Study the drawing (mm; zero at the part's minimum x, y, z) and answer. A direction names the side the tool comes from. Give positions to 0.01 mm unless a question says otherwise; leave off trailing zeros. Order: outer loops, then holes, each group sorted by start corner. A loop starts at its lowest first (then second) coordinate and runs counter-clockwise, first axis right, second up. Notation, with made-up numbers: (41, -37) - (83, -37) arc R10 cw to (83, -25) - close; hole circle Ø8 at (34, 83.5). An arc over 180 degrees is marked (long way). Use CSV: the item, a comma, the result in double quotes.
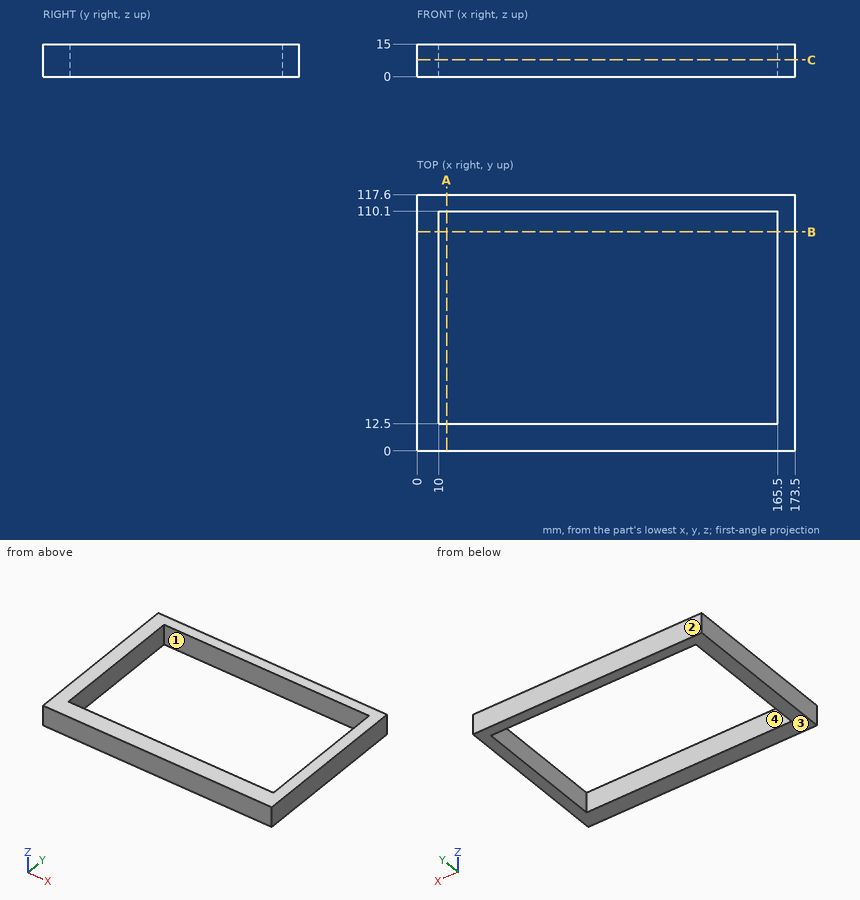
Item 1: Which of the six approach directions +Z, -Z, +X, -X, +Y, -Y give full straight-line access (tool end or side, diameter ignored) to the marked faces 3 and 4?
Taken from the geometry:
face 3,"-Z, +X, -X, +Y, -Y"
face 4,"+Z, -Z"
Item 2: The part is cut by section A-A (x = 13.5). Give the vertices of the cut face in (y, z).
Taken from the geometry:
outline,"(0, 0) - (12.5, 0) - (12.5, 15) - (0, 15) - close; (110.1, 0) - (117.6, 0) - (117.6, 15) - (110.1, 15) - close"
Item 3: The part is cut by section C-C (z = 7.75). Give the vertices of the cut face in (x, y), and give its area (3 significant figures).
Taken from the geometry:
outline,"(0, 0) - (173.5, 0) - (173.5, 117.6) - (0, 117.6) - close; hole (10, 12.5) - (165.5, 12.5) - (165.5, 110.1) - (10, 110.1) - close"
area,"5,230 mm^2"
Item 4: This flat-tipped pin is pushed along its axis until it touches: pin 1 (12 mm diameter, centred on x = 18, y = 89, fed in from +Z) (3 decimals). Where does it stop, or does it pass through?
Taken from the geometry:
pin 1,"through"
Item 5: Find the intervals of material crossed by line 1 along Y through (x, z) = (74, 13.25); line 2 along X through (y, z) = (20.5, 9.5), in increasing order.
Taken from the geometry:
line 1,"0 to 12.5, 110.1 to 117.6"
line 2,"0 to 10, 165.5 to 173.5"
Item 6: The part is cut by section B-B (y = 100.5). Give the vertices of the cut face in (x, z), and give its area (3 significant figures).
Taken from the geometry:
outline,"(0, 0) - (10, 0) - (10, 15) - (0, 15) - close; (165.5, 0) - (173.5, 0) - (173.5, 15) - (165.5, 15) - close"
area,"270 mm^2"
Item 7: The mould has two halves that part along X. Classify the marked faces 1 and 2: +X half, -X half, draft (parallel to the pull), parting line (faces both ways), or undercut.
Taken from the geometry:
face 1,"undercut"
face 2,"draft"
